from build123d import *

# Parameters (mm, degrees)
SKETCH1_W     = 142
SKETCH1_H     = 56
SKETCH1_W_2   = 138
SKETCH1_H_2   = 52
PROFILE_DEPTH = 93
SKETCH2_W     = 138
SKETCH2_H     = 52
BACK_DEPTH    = 2


with BuildPart() as part:
    # Sketch1 → Profile (new body)
    with BuildSketch(Plane.XY):
        with Locations((71, 28)):
            Rectangle(SKETCH1_W, SKETCH1_H)
        with Locations((71, 28)):
            Rectangle(SKETCH1_W_2, SKETCH1_H_2, mode=Mode.SUBTRACT)
    extrude(amount=PROFILE_DEPTH)

    # Sketch2 → Back (add)
    with BuildSketch(Plane.XY):
        with Locations((71, 28)):
            Rectangle(SKETCH2_W, SKETCH2_H)
    extrude(amount=BACK_DEPTH)


solid = part.part
Geometry check sheet. Reference: the model listing, model coordinates, mm. A direction names the side the tool comes from. Give positions to 0.01 mm unless a question says otherwise; leave off trailing zeros. Loops run counter-clockwise (first coordinate to the right, second up) from the corner with the lowest first, then second, coordinate; pieces in that order, holes last.
(1) Depth check by flat-ended pin: pin 1 Ø15.5 at (x, y) = (72, 23.5) entering from +Z. Enter the tip coordinate at first touch or a pass-through.
From the geometry:
pin 1: stops at z = 2
(2) Section check B-B on y = 52. Record the cut outline in (x, z), then the cut area to 3 significant figures.
From the geometry:
outline: (0, 0) - (142, 0) - (142, 93) - (140, 93) - (140, 2) - (2, 2) - (2, 93) - (0, 93) - close
area: 648 mm2
(3) Set-up check for faces 1 (the flat face through (140, 28, 47)), 2 (the flat face through (70, 0, 46)): record each of +Z, -Z, +X, -X, +Y, -Y from which the full face is reachable in a straight line by a thin tool's end or side.
From the geometry:
face 1: +Z
face 2: +Z, -Z, +X, -X, -Y
(4) Section check C-C on x = 35. Record the cut outline in (y, z).
From the geometry:
outline: (0, 0) - (56, 0) - (56, 93) - (54, 93) - (54, 2) - (2, 2) - (2, 93) - (0, 93) - close
(5) Release check for a two-part mould opening along Y. For faces 3 (the flat face through (70, 56, 46)), 4 (the flat face through (70, 28, 2)), 5 (the flat face through (71, 55, 93)) record: released by +Y, released by -Y, zero draft, split by the parting line, or undercut.
From the geometry:
face 3: released by +Y
face 4: undercut
face 5: zero draft
(6) Section check A-A on z = 24. Record the cut outline in (x, y).
From the geometry:
outline: (0, 0) - (142, 0) - (142, 56) - (0, 56) - close; hole (2, 2) - (140, 2) - (140, 54) - (2, 54) - close
(7) Thickness scan on L1, parallel to Y at x = 113.5, z = 65; L2, parallel to X at y = 38, z = 63.5; L3, parallel to Z at x = 126, y = 11.5. Record the ranges inside material, lowest first.
From the geometry:
L1: y = 0 to 2, 54 to 56
L2: x = 0 to 2, 140 to 142
L3: z = 0 to 2
